from build123d import *

# Parameters (mm, degrees)
F1_DEPTH = 15
F2_R     = 2.75
F3_R     = 2
F5_DEPTH = 2.5
F6_SIZE2 = 10
F6_SIZE  = 2.5
F7_R     = 2.75
F8_DEPTH = 3
F9_R     = 0.5


with BuildPart() as f1:
    # F0 (on Right) → F1 (new body)
    with BuildSketch(Plane.YZ):
        Polygon((-17, 0), (0, 0), (0, 25), (-1, 25), (-1, 2.5), (-17, 2.5), align=None)
    extrude(amount=F1_DEPTH)

    # F2
    f2_edges = [f1.edges().sort_by_distance(p)[0] for p in [
        (7.5, -1, 2.5),
    ]]
    fillet(f2_edges, radius=F2_R)

    # F3
    f3_edges = [f1.edges().sort_by_distance(p)[0] for p in [
        (15, -17, 1.25),
        (0, -17, 1.25),
    ]]
    fillet(f3_edges, radius=F3_R)

    # F4 (on face) → F5 (cut)
    with BuildSketch(Plane.XY.offset(2.5)):
        with BuildLine():
            Line((9.5, -9.525), (9.5, -6.525))
            ThreePointArc((9.5, -6.525), (8.9142135624, -5.1107864376), (7.5, -4.525))
            ThreePointArc((7.5, -4.525), (6.0857864376, -5.1107864376), (5.5, -6.525))
            Line((5.5, -6.525), (5.5, -9.525))
            ThreePointArc((5.5, -9.525), (6.0857864376, -10.9392135624), (7.5, -11.525))
            ThreePointArc((7.5, -11.525), (8.9142135624, -10.9392135624), (9.5, -9.525))
        make_face()
    extrude(amount=-F5_DEPTH, mode=Mode.SUBTRACT)

    # F6
    f6_edges = [f1.edges().sort_by_distance(p)[0] for p in [
        (15, -0.5, 25),
        (0, -0.5, 25),
    ]]
    f6_side = f1.faces().sort_by_distance((7.5, -0.5, 25))[0]
    chamfer(f6_edges, length=F6_SIZE, length2=F6_SIZE2, reference=f6_side)

    # F7 (on face) → F8 (cut)
    with BuildSketch(Plane.XZ.offset(1)):
        with Locations((7.5, 19)):
            Circle(F7_R)
    extrude(amount=-F8_DEPTH, mode=Mode.SUBTRACT)

    # F9
    f9_edges = [f1.edges().sort_by_distance(p)[0] for p in [
        (12.5, -0.5, 25),
        (2.5, -0.5, 25),
    ]]
    fillet(f9_edges, radius=F9_R)


solid = f1.part
Work out the finished part from the listing and answer in its coordinate system (mm). A direction names the side the tool comes from. Give positions to 0.01 mm unless a question says otherwise; leave off trailing zeros. Write each loop counter-clockwise with the first axis right and the second up, starting at its lowest first coordinate (ties: lowest second). Pieces come first, ordered by that corner, then holes.
Q1. The part is cut by section C-C on x = 13.75. Give the vertices of the cut face in (y, z).
Answer:
outline: (-16.85, 0) - (0, 0) - (0, 20) - (-1, 20) - (-1, 5.25) arc R2.75 cw to (-3.75, 2.5) - (-16.85, 2.5) - close
Q2. The part is cut by section B-B on z = 19. Give the vertices of the cut face in (x, y).
Answer:
outline: (1, -1) - (4.75, -1) - (4.75, 0) - (1, 0) - close; (10.25, -1) - (14, -1) - (14, 0) - (10.25, 0) - close
Q3. Straight lines are drawn through the part: L1, parallel to Z at x = 7.5, y = -0.2; L2, parallel to Z at x = 1, y = -15.5; L3, parallel to Y at x = 13.5, z = 17.5. For each, find the intervals that lie inside material, in ascending order.
Answer:
L1: z = 0 to 16.25, 21.75 to 25
L2: z = 0 to 2.5
L3: y = -1 to 0
Q4. Given pin 1 (2 mm diameter, centred on x = 2.5, z = 17, fed in from -Y); pin 2 (4 mm diameter, centred on x = 8, y = -10, fed in from +Z); pin 3 (5 mm diameter, centred on x = 7.5, z = 19, fed in from +Y), each flat-ended and moving along its own axis, determine where each tip first touches the part or whether it passes through.
Answer:
pin 1: stops at y = -1
pin 2: stops at z = 2.5
pin 3: passes through
Q5. A tool of negligible diameter and unlimited length cuts with its end or side. For faces 4 (the face through (7, -1, 15)), 5 (the face through (5.5, -8, 1)), 6 (the face through (7, 0, 12)), from which of +Z, -Z, +X, -X, +Y, -Y can it reach the whole face along a straight path? Write none if from no direction.
Answer:
face 4: +Z, +X, -X, -Y
face 5: +Z, -Z
face 6: +Z, -Z, +X, -X, +Y
Q6. The part is cut by section A-A on y = -8.5. Give the vertices of the cut face in (x, z).
Answer:
outline: (0, 0) - (5.5, 0) - (5.5, 2.5) - (0, 2.5) - close; (9.5, 0) - (15, 0) - (15, 2.5) - (9.5, 2.5) - close
Q7. For a pull along X with two mould halves and no side action, classify faces 1 (the face through (7, -12, 2.5)), 2 (the face through (15, -5, 2)), 3 (the face through (9.5, -8, 1)) as released by +X, released by -X, zero draft, split by the parting line, or undercut.
Answer:
face 1: zero draft
face 2: released by +X
face 3: undercut
Q8. The part is cut by section D-D on x = 6.5. Give the vertices of the cut face in (y, z).
Answer:
outline: (-17, 0) - (-11.26, 0) - (-11.26, 2.5) - (-17, 2.5) - close; (-4.79, 0) - (0, 0) - (0, 16.44) - (-1, 16.44) - (-1, 5.25) arc R2.75 cw to (-3.75, 2.5) - (-4.79, 2.5) - close; (-1, 21.56) - (0, 21.56) - (0, 25) - (-1, 25) - close
